Build history of the part. All positions in model axes, mm. A direction names the side the tool comes from. Round coordinates to 2 decimals unless told otherwise and drop trailing zeros. Write each loop counter-clockwise with the first axis right and the second up, starting at its lowest first coordinate (ties: lowest second). Pieces come first, ordered by that corner, then holes. Notation, with made-up numbers: (-21, 41) -> (-3, 41) arc R27 ccw to (-3, 77) -> close; hole circle Ø6 at (4.5, -39). An arc over 180 degrees is marked (long way). Answer in a Markdown table with one row per item.
```python
from build123d import *

# Parameters (mm, degrees)
ESQUISSE1_R                  = 1.6
BOSS_EXTRU_1_DEPTH           = 8
ESQUISSE2_R                  = 1
ENL_V_MAT_EXTRU_1_DEPTH      = 8
R_P_TITION_LIN_AIRE1_COUNT   = 7
R_P_TITION_LIN_AIRE1_PITCH   = 5
ESQUISSE3_W                  = 63.02569825
ESQUISSE3_H                  = 22.447508966
ESQUISSE3_R                  = 6
ENL_V_MAT_EXTRU_2_DEPTH      = 2
ESQUISSE4_W                  = 65.150237544
ESQUISSE4_H                  = 23.585889013
ESQUISSE4_R                  = 4.65
ENL_V_MAT_EXTRU_3_DEPTH      = 1
ESQUISSE5_R                  = 2.75
ENL_V_MAT_EXTRU_4_DEPTH      = 1
CHANFREIN1_SIZE              = 1
ESQUISSE6_R                  = 4
ENL_V_MAT_EXTRU_5_DEPTH      = 5
BOSS_EXTRU_2_DEPTH           = 5
R_P_TITION_CIRCULAIRE1_COUNT = 24
ESCALA2_SCALE                = 0.7
ESCALA5_SCALE                = 0.8
ESCALA6_SCALE                = 0.9
ESCALA7_SCALE                = 0.9
ESCALA8_SCALE                = 1.05
ESCALA9_SCALE                = 1.2
ESCALA11_SCALE               = 0.8


with BuildPart() as part:
    # Esquisse1 → Boss.-Extru.1 (new body)
    with BuildSketch(Plane(origin=(0, 0, 0), x_dir=(1, 0, 0), z_dir=(0, 1, 0))):
        with BuildLine():
            Line((0.874233129, -7.448873501), (41.070552147, -2.731253617))
            ThreePointArc((41.070552147, -2.731253617), (43.5, 0), (41.070552147, 2.731253617))
            Line((41.070552147, 2.731253617), (0.874233129, 7.448873501))
            ThreePointArc((0.874233129, 7.448873501), (-7.5, 0), (0.874233129, -7.448873501))
        make_face()
        with Locations(Location((0, 0, 0), (0, 0, 270))):
            Circle(ESQUISSE1_R, mode=Mode.SUBTRACT)
    extrude(amount=BOSS_EXTRU_1_DEPTH)

    # Esquisse2 → Enlèv. mat.-Extru.1 (cut)
    with BuildSketch(Plane(origin=(0, 8, 0), x_dir=(1, 0, 0), z_dir=(0, 1, 0))):
        with Locations(Location((9.5, 0, 0), (0, 0, 270))):
            Circle(ESQUISSE2_R)
    enl_v_mat_extru_1 = extrude(amount=-ENL_V_MAT_EXTRU_1_DEPTH, mode=Mode.SUBTRACT)

    # Répétition linéaire1: Enlèv. mat.-Extru.1 ×7
    with Locations(*[(i * R_P_TITION_LIN_AIRE1_PITCH, 0, 0) for i in range(1, R_P_TITION_LIN_AIRE1_COUNT)]):
        add(enl_v_mat_extru_1, mode=Mode.SUBTRACT)

    # Esquisse3 → Enlèv. mat.-Extru.2 (cut)
    with BuildSketch(Plane(origin=(0, 8, 0), x_dir=(1, 0, 0), z_dir=(0, 1, 0))):
        with Locations((18.729808022, -1.006570064)):
            Rectangle(ESQUISSE3_W, ESQUISSE3_H)
        with Locations(Location((0, 0, 0), (0, 0, 270))):
            Circle(ESQUISSE3_R, mode=Mode.SUBTRACT)
    extrude(amount=-ENL_V_MAT_EXTRU_2_DEPTH, mode=Mode.SUBTRACT)

    # Esquisse4 → Enlèv. mat.-Extru.3 (cut)
    with BuildSketch(Plane.XZ):
        with Locations((19.098187779, 0.565848797)):
            Rectangle(ESQUISSE4_W, ESQUISSE4_H)
        with Locations(Location((0, 0, 0), (0, 0, 270))):
            Circle(ESQUISSE4_R, mode=Mode.SUBTRACT)
    extrude(amount=-ENL_V_MAT_EXTRU_3_DEPTH, mode=Mode.SUBTRACT)

    # Esquisse5 → Enlèv. mat.-Extru.4 (cut)
    with BuildSketch(Plane.XZ):
        with Locations(Location((0, 0, 0), (0, 0, 270))):
            Circle(ESQUISSE5_R)
    extrude(amount=-ENL_V_MAT_EXTRU_4_DEPTH, mode=Mode.SUBTRACT)

    # Chanfrein1
    chanfrein1_edges = [part.edges().sort_by_distance(p)[0] for p in [
        (0, 1, 4.65),
    ]]
    chamfer(chanfrein1_edges, length=CHANFREIN1_SIZE - 0.0001)  # a hair under: the kernel refuses the full size

    # Esquisse6 → Enlèv. mat.-Extru.5 (cut)
    with BuildSketch(Plane(origin=(0, 8, 0), x_dir=(1, 0, 0), z_dir=(0, 1, 0))):
        with Locations(Location((0, 0, 0), (0, 0, 270))):
            Circle(ESQUISSE6_R)
    extrude(amount=-ENL_V_MAT_EXTRU_5_DEPTH, mode=Mode.SUBTRACT)

    # Esquisse7 → Boss.-Extru.2 (add)
    with BuildSketch(Plane(origin=(0, 8, 0), x_dir=(1, 0, 0), z_dir=(0, 1, 0))):
        Polygon((0.3, -4), (0.139230485, -3.4), (-0.139230485, -3.4), (-0.3, -4), align=None)
    boss_extru_2 = extrude(amount=-BOSS_EXTRU_2_DEPTH)

    # Répétition circulaire1: Boss.-Extru.2 ×24 about axis
    r_p_tition_circulaire1_axis = Axis((0, 0, 0), (0, 1, 0))
    for i in range(1, R_P_TITION_CIRCULAIRE1_COUNT):
        add(boss_extru_2.rotate(r_p_tition_circulaire1_axis, i * 360 / R_P_TITION_CIRCULAIRE1_COUNT))


with BuildPart() as part_1:
    # Escala2: scaled about (13.607866543, 3.578266839, 0)
    add(part.part.scale(ESCALA2_SCALE).moved(Location((4.082359963, 1.073480052, 0))))


with BuildPart() as part_2:
    # Escala5: scaled about (13.607866543, 3.578266839, 0)
    add(part_1.part.scale(ESCALA5_SCALE).moved(Location((2.721573309, 0.715653368, 0))))


with BuildPart() as part_3:
    # Escala6: scaled about (13.607866543, 3.578266839, 0)
    add(part_2.part.scale(ESCALA6_SCALE).moved(Location((1.360786654, 0.357826684, 0))))


with BuildPart() as part_4:
    # Escala7: scaled about (13.607866543, 3.578266839, 0)
    add(part_3.part.scale(ESCALA7_SCALE).moved(Location((1.360786654, 0.357826684, 0))))


with BuildPart() as part_5:
    # Escala8: scaled about (13.607866543, 3.578266839, 0)
    add(part_4.part.scale(ESCALA8_SCALE).moved(Location((-0.680393327, -0.178913342, 0))))


with BuildPart() as part_6:
    # Escala9: scaled about (13.607866543, 3.578266839, 0)
    add(part_5.part.scale(ESCALA9_SCALE).moved(Location((-2.721573309, -0.715653368, 0))))


with BuildPart() as part_7:
    # Escala11: scaled about (13.607866543, 3.578266839, 0)
    add(part_6.part.scale(ESCALA11_SCALE).moved(Location((2.721573309, 0.715653368, 0))))


solid = part_7.part
```
Q1. Which spindle directions (+Z, -Z, +X, -X, +Y, -Y) get a long thin tool onto all of the face, cutting with end or side? Do faces 5 (the cylindrical face through (6.672, 2.85, -0.159)), 6 (the flat face through (7, 2.399, -1)), 7 (the cylindrical face through (4.708, 5.149, -0.595)). Say none if no direction does.
A:
| item | result |
|---|---|
| face 5 | +Y, -Y |
| face 6 | -Y |
| face 7 | +Y |
Q2. Saw through at B-B on y = 2.7. State how many separate pieces and enclosed holes the cut face has, plus the area to 3 significant figures.
A:
| item | result |
|---|---|
| separate pieces | 1 |
| enclosed holes | 8 |
| area | 103 mm² |
Q3. Drop flat-ended pins along their axis: P1, Ø4, axis at x = 17, z = 1, coming from the +Y side; P2, Ø2, axis at x = 21.5, z = -2.5, coming from the -Y side; P3, Ø1.1, axis at x = 8, z = 0.5, coming from the +Y side. Give the stop position or say it passes through.
A:
| item | result |
|---|---|
| P1 | y = 4.69 |
| P2 | y = 2.4 |
| P3 | y = 3.31 |
Q4. Saw through at A-A on x = 11.5. Write the cut outline in (y, z).
A:
| item | result |
|---|---|
| outline | (2.4, -2.97) -> (4.69, -2.97) -> (4.69, -0.4) -> (2.4, -0.4) -> close; (2.4, 0.4) -> (4.69, 0.4) -> (4.69, 2.97) -> (2.4, 2.97) -> close |
Q5. Wall check: line 1 (Y direction, x = 5.75, z = -2.5); line 2 (X direction, y = 2.15, z = 0); line 3 (Z direction, x = 25.75, y = 2.8). Give the ranges that are in metal, low to high. Write a range as [from, to].
A:
| item | result |
|---|---|
| line 1 | [2.4, 4.69] |
| line 2 | [5.05, 6.13], [8.64, 9.72] |
| line 3 | [-1.3, -0.34], [0.34, 1.3] |
Q6. Two-plate mould, pull along Z, no slides. Class faces 1 (the cylindrical face through (8.633, 2.168, 0.164)), 2 (the cylindrical face through (27.275, 3.526, 0.026)), 3 (the flat face through (15, 4.686, 0)), 4 (the cylindrical face through (25.83, 3.56, 0.25)): released by +Z, released by -Z, zero draft, split by the parting line, or undercut.
A:
| item | result |
|---|---|
| face 1 | undercut |
| face 2 | split by the parting line |
| face 3 | zero draft |
| face 4 | undercut |
Q7. Saw through at C-C on x = 15.5. Write the cut outline in (y, z).
A:
| item | result |
|---|---|
| outline | (2.4, -2.5) -> (4.69, -2.5) -> (4.69, 2.5) -> (2.4, 2.5) -> close |
